For this review, take the finished solid that the model builds, in its own axes (mm). A direction names the side the tool comes from. Coordinates: 2 decimals unless noted, no trailing zeros. Order: outer loops, then holes, each group sorted by start corner. A loop starts at its lowest first (then second) coordinate and runs counter-clockwise, first axis right, second up. Notation, with made-up numbers: (32.5, 2) -> (89.5, 2) arc R20 cw to (89.5, 28) -> close; hole circle Ø10 at (-17, 3.25). An arc over 180 degrees is marked (long way). Write item = value, one per line. Start each with the question number.
1) Draft analysis for pull direction Z (two halves, no side actions). For faces 4 (the face through (38.79, -38.97, 1.01)), 5 (the face through (-46.737, -14.718, 12.423)), 6 (the face through (-4, 46, 25)), state which applies: +Z half, -Z half, draft (parallel to the pull), parting line (faces both ways), or undercut.
2) Consider section B-B on y = 0. Give the boundary of the cut face in (x, z).
3) Wall thickness on probe 1 along Y at (x, z) = (0, 10); probe 2 along X at (y, z) = (27, 23.5); probe 3 along Y at (x, z) = (3.5, 11.75): over which ranges is each line inside the solid? List them lowest first. Write a range as [from, to].
4) Insertion check: pin 1 Ø8 at (x, y) = (29, 28.5) entering from +Z; pin 2 Ø10 at (x, z) = (-4, 12) entering from -Y; pin 3 Ø0.6 at (y, z) = (27.5, 0.5) entering from +X. Each pin has a flat end and moves straight along its axis. Give the tip position at first contact, or say it passes through.
5) Machinability: for faces 1 (the face through (0, -3, 2)), 2 (the face through (21.76, -15.45, 0.99)), 3 (the face through (-38, 38, 2)), which of the approach directions +Z, -Z, +X, -X, +Y, -Y give a long, thin tool a straight path to every point of the face, cutting with its end or side? Answer none if there is none.
6) Consider section A-A on x = 0. Give the boundary of the cut face in (y, z).
7) Consider section D-D on x = 41. State how many separate pieces and enclosed holes the cut face has, and give its area (3 significant figures).
8) Consider section C-C on z = 21.75. Give the boundary of the cut face in (x, y), and give its area (3 significant figures).
from build123d import *

# Parameters (mm, degrees)
CROQUIS1_R              = 10
SALIENTE_EXTRUIR2_DEPTH = 2
CROQUIS1_5_R            = 50
CROQUIS1_5_R_2          = 44
SALIENTE_EXTRUIR3_DEPTH = 25
CHAFL_N1_SIZE           = 2
CROQUIS3_R              = 3
CORTAR_EXTRUIR1_DEPTH   = 25


with BuildPart() as part:
    # Croquis1 → Saliente-Extruir2 (new body)
    with BuildSketch(Plane.XY):
        with BuildLine():
            Line((-46, 46), (-46, 19.595917942))
            ThreePointArc((-46, 19.595917942), (-35.355339059, 35.355339059), (-19.595917942, 46))
            Line((-19.595917942, 46), (-46, 46))
        make_face()
        with BuildLine():
            ThreePointArc((-19.595917942, -46), (-35.355339059, -35.355339059), (-46, -19.595917942))
            Line((-46, -19.595917942), (-46, -46))
            Line((-46, -46), (-19.595917942, -46))
        make_face()
        with BuildLine():
            ThreePointArc((46, -19.595917942), (35.355339059, -35.355339059), (19.595917942, -46))
            Line((19.595917942, -46), (46, -46))
            Line((46, -46), (46, -19.595917942))
        make_face()
        with BuildLine():
            Line((46, 46), (19.595917942, 46))
            ThreePointArc((19.595917942, 46), (35.355339059, 35.355339059), (46, 19.595917942))
            Line((46, 19.595917942), (46, 46))
        make_face()
        Circle(CROQUIS1_R)
        with BuildLine():
            Line((-2.5, 43.928919859), (-2.5, 9.682458366))
            ThreePointArc((-2.5, 9.682458366), (0, 10), (2.5, 9.682458366))
            Line((2.5, 9.682458366), (2.5, 43.928919859))
            ThreePointArc((2.5, 43.928919859), (0, 44), (-2.5, 43.928919859))
        make_face()
        with BuildLine():
            ThreePointArc((-7.135254916, -7.006292692), (-8.660254038, -5), (-9.635254916, -2.676165673))
            Line((-9.635254916, -2.676165673), (-39.293560559, -19.79939642))
            ThreePointArc((-39.293560559, -19.79939642), (-38.105117767, -22), (-36.793560559, -24.129523439))
            Line((-36.793560559, -24.129523439), (-7.135254916, -7.006292692))
        make_face()
        with BuildLine():
            Line((39.293560559, -19.79939642), (9.635254916, -2.676165673))
            ThreePointArc((9.635254916, -2.676165673), (8.660254038, -5), (7.135254916, -7.006292692))
            Line((7.135254916, -7.006292692), (36.793560559, -24.129523439))
            ThreePointArc((36.793560559, -24.129523439), (38.105117767, -22), (39.293560559, -19.79939642))
        make_face()
    extrude(amount=SALIENTE_EXTRUIR2_DEPTH)

    # Croquis1_5 → Saliente-Extruir3 (add)
    with BuildSketch(Plane.XY):
        with Locations(Location((0, 0, 0), (0, 0, 156.926081934))):
            Circle(CROQUIS1_5_R)
        with Locations(Location((0, 0, 0), (0, 0, 206.742803839))):
            Circle(CROQUIS1_5_R_2, mode=Mode.SUBTRACT)
    extrude(amount=SALIENTE_EXTRUIR3_DEPTH)

    # Croquis2 → Cortar-Revoluci_n1 (revolve, cut)
    with BuildSketch(Plane(origin=(0, 0, 0), x_dir=(0, 0, -1), z_dir=(1, 0, 0)), mode=Mode.PRIVATE) as cortar_revoluci_n1_sk:
        Polygon((-5, 50), (-20, 50), (-18, 49), (-7, 49), align=None)
    revolve(cortar_revoluci_n1_sk.sketch.rotate(Axis((0, 0, -1.25), (0, 0, 1)), 90), axis=Axis((0, 0, -1.25), (0, 0, 1)), mode=Mode.SUBTRACT)

    # Chafl_n1
    chafl_n1_edges = [part.edges().sort_by_distance(p)[0] for p in [
        (39.293560559, 19.79939642, 25),
    ]]
    chamfer(chafl_n1_edges, length=CHAFL_N1_SIZE)

    # Croquis3 → Cortar-Extruir1 (cut)
    with BuildSketch(Plane.XY.offset(2)):
        with Locations((-41, 41)):
            Circle(CROQUIS3_R)
        with Locations((-41, -41)):
            Circle(CROQUIS3_R)
        with Locations((41, 41)):
            Circle(CROQUIS3_R)
        with Locations((41, -41)):
            Circle(CROQUIS3_R)
    extrude(amount=-CORTAR_EXTRUIR1_DEPTH, mode=Mode.SUBTRACT)


solid = part.part
Answer sheet:
q1.face_4 = draft
q1.face_5 = undercut
q1.face_6 = +Z half
q2.outline = (-50, 0) -> (-44, 0) -> (-44, 23) -> (-46, 25) -> (-50, 25) -> (-50, 20) -> (-49, 18) -> (-49, 7) -> (-50, 5) -> close; (-10, 0) -> (10, 0) -> (10, 2) -> (-10, 2) -> close; (44, 0) -> (50, 0) -> (50, 5) -> (49, 7) -> (49, 18) -> (50, 20) -> (50, 25) -> (46, 25) -> (44, 23) -> close
q3.probe_1 = [-49, -44], [44, 49]
q3.probe_2 = [-42.08, -35.37], [35.37, 42.08]
q3.probe_3 = [-48.87, -43.86], [43.86, 48.87]
q4.pin_1 = 23.66
q4.pin_2 = -49
q4.pin_3 = 46
q5.face_1 = +Z
q5.face_2 = +Z, -Z
q5.face_3 = +Z, -X, +Y
q6.outline = (-50, 0) -> (-44, 0) -> (-44, 23) -> (-46, 25) -> (-50, 25) -> (-50, 20) -> (-49, 18) -> (-49, 7) -> (-50, 5) -> close; (-10, 0) -> (50, 0) -> (50, 5) -> (49, 7) -> (49, 18) -> (50, 20) -> (50, 25) -> (46, 25) -> (44, 23) -> (44, 2) -> (-10, 2) -> close
q7.separate_pieces = 4
q7.enclosed_holes = 0
q7.area = 621 mm2
q8.outline = circle Ø100 at (0, 0); hole circle Ø88 at (0, 0)
q8.area = 1,770 mm2
